For this review, use the dimensioned drawing (mm, ordinates from the lowest corner) and the shaded views. A direction names the side the tool comes from. Give positions to 0.01 mm unless a question says otherwise; leave off trailing zeros. Order: outer loops, then holes, each group sorted by start corner. A loop starts at its lowest first (then second) coordinate and runs counter-clockwise, first axis right, second up. Notation, with made-up numbers: (-33.5, 34) -> (-2.5, 34) arc R36 ccw to (-2.5, 70) -> close; hole circle Ø7 at (40.5, -7). An arc over 180 degrees is marked (long way). Answer as a JSON object with one key per item and string values. Group by question number.
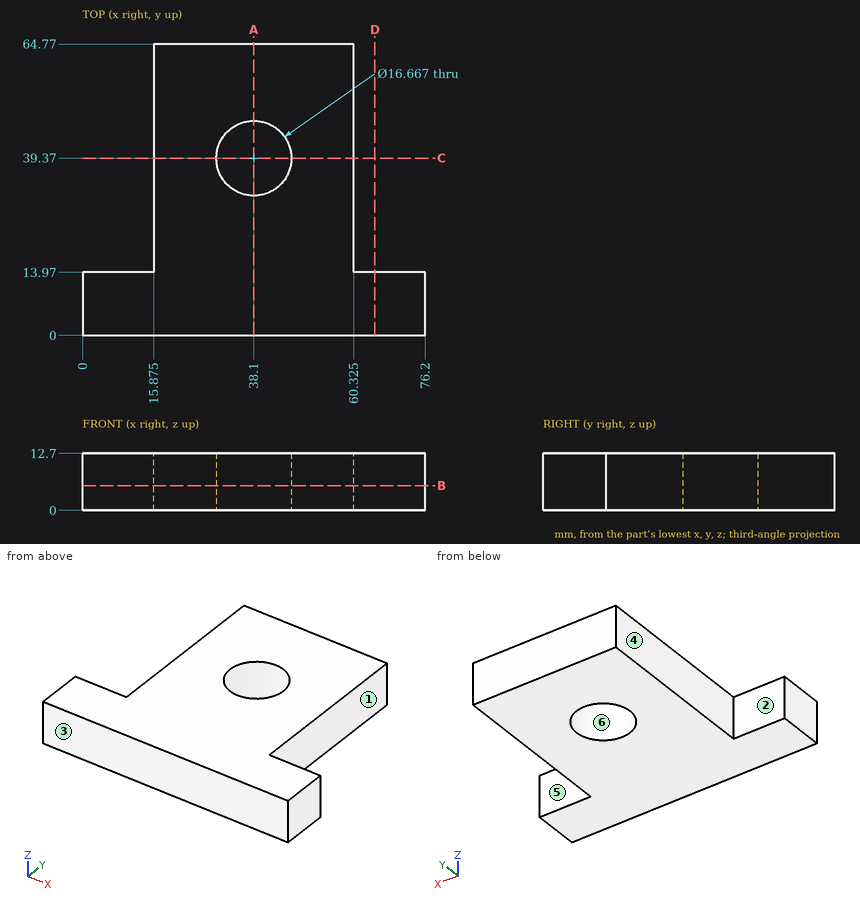
1. Take a section at C-C on y = 39.37. Give the boundary of the cut face in (x, z) (1 decimal).
2. For pin 1 (4 mm diameter, centred on y = 42.5, z = 3.5, fed in from +X) (1 decimal); pin 2 (6.5 mm diameter, centred on x = 6.5, z = 8, fed in from +Y); pin 3 (3 mm diameter, centred on y = 27.5, z = 5.5, fed in from -X) (1 decimal), all flat-tipped, find the tip position at first contact; note any pin that passes through.
3. Machinability: for the marked faces 1, 2 and 3, which of the approach directions +Z, -Z, +X, -X, +Y, -Y give a long, thin tool a straight path to every point of the face, cutting with its end or side? Answer none if there is none.
4. Take a section at B-B on z = 5.5. Give the boundary of the cut face in (x, y) (1 decimal).
5. Take a section at A-A on x = 38.1. Give the boundary of the cut face in (y, z).
6. Draft analysis for pull direction X (two halves, no side actions). For the marked faces 4, 5 and 6, state which applies: pulls with the +X half, pulls with the -X half, needs draft (parallel to the pull), parting line crosses it, or undercut.
7. Take a section at D-D on x = 65. Give the boundary of the cut face in (y, z).
8. For probe 1 along Y at (x, z) = (38.5, 4.5) (1 decimal); probe 2 along X at (y, z) = (15, 0.5) (1 decimal); probe 3 along X at (y, z) = (34, 12.25) (1 decimal), list the stretches that pass through material, from the lowest coordinate up. Write a range as [from, to].
Checks:
{
 "1": {"outline": "(15.9, 0) -> (29.8, 0) -> (29.8, 12.7) -> (15.9, 12.7) -> close; (46.4, 0) -> (60.3, 0) -> (60.3, 12.7) -> (46.4, 12.7) -> close"},
 "2": {"pin 1": "stops at x = 60.3", "pin 2": "stops at y = 13.97", "pin 3": "stops at x = 15.9"},
 "3": {"face 1": "+Z, -Z, +X, +Y", "face 2": "+Z, -Z, -X, +Y", "face 3": "+Z, -Z, +X, -X, -Y"},
 "4": {"outline": "(0, 0) -> (76.2, 0) -> (76.2, 14) -> (60.3, 14) -> (60.3, 64.8) -> (15.9, 64.8) -> (15.9, 14) -> (0, 14) -> close; hole circle Ø16.7 at (38.1, 39.4)"},
 "5": {"outline": "(0, 0) -> (31.04, 0) -> (31.04, 12.7) -> (0, 12.7) -> close; (47.7, 0) -> (64.77, 0) -> (64.77, 12.7) -> (47.7, 12.7) -> close"},
 "6": {"face 4": "pulls with the -X half", "face 5": "needs draft", "face 6": "undercut"},
 "7": {"outline": "(0, 0) -> (13.97, 0) -> (13.97, 12.7) -> (0, 12.7) -> close"},
 "8": {"probe 1": "y = [0, 31], [47.7, 64.8]", "probe 2": "x = [15.9, 60.3]", "probe 3": "x = [15.9, 31.7], [44.5, 60.3]"}
}
